from build123d import *

# Parameters (mm, degrees)
SKETCH1_W           = 72.136
SKETCH1_H           = 97.536
BOSS_EXTRUDE1_DEPTH = 6.35
CUT_EXTRUDE4_REACH  = 123.479
SKETCH12_R          = 2.54
SKETCH13_R          = 1.27
CUT_EXTRUDE5_DEPTH  = 3.81


with BuildPart() as part:
    # Sketch1 → Boss-Extrude1 (new body)
    with BuildSketch(Plane.XY):
        with Locations((36.068, -48.768)):
            Rectangle(SKETCH1_W, SKETCH1_H)
    extrude(amount=BOSS_EXTRUDE1_DEPTH)

    # Sketch12 → Cut-Extrude4 (cut, up to next)
    with BuildSketch(Plane.XY.offset(6.35), mode=Mode.PRIVATE) as cut_extrude4_sk1:
        with Locations((3.048, -3.048)):
            Circle(SKETCH12_R)
    cut_extrude4_tool1 = extrude(cut_extrude4_sk1.sketch, amount=-CUT_EXTRUDE4_REACH, mode=Mode.PRIVATE) & part.part
    # Sketch12 → Cut-Extrude4 (cut, up to next)
    with BuildSketch(Plane.XY.offset(6.35), mode=Mode.PRIVATE) as cut_extrude4_sk2:
        with Locations((69.088, -3.048)):
            Circle(SKETCH12_R)
    cut_extrude4_tool2 = extrude(cut_extrude4_sk2.sketch, amount=-CUT_EXTRUDE4_REACH, mode=Mode.PRIVATE) & part.part
    # Sketch12 → Cut-Extrude4 (cut, up to next)
    with BuildSketch(Plane.XY.offset(6.35), mode=Mode.PRIVATE) as cut_extrude4_sk3:
        with Locations((69.088, -94.488)):
            Circle(SKETCH12_R)
    cut_extrude4_tool3 = extrude(cut_extrude4_sk3.sketch, amount=-CUT_EXTRUDE4_REACH, mode=Mode.PRIVATE) & part.part
    # Sketch12 → Cut-Extrude4 (cut, up to next)
    with BuildSketch(Plane.XY.offset(6.35), mode=Mode.PRIVATE) as cut_extrude4_sk4:
        with Locations((3.048, -94.488)):
            Circle(SKETCH12_R)
    cut_extrude4_tool4 = extrude(cut_extrude4_sk4.sketch, amount=-CUT_EXTRUDE4_REACH, mode=Mode.PRIVATE) & part.part
    add(cut_extrude4_tool1.solids().sort_by_distance((3.048, -3.048, 6.35))[0], mode=Mode.SUBTRACT)
    add(cut_extrude4_tool2.solids().sort_by_distance((69.088, -3.048, 6.35))[0], mode=Mode.SUBTRACT)
    add(cut_extrude4_tool3.solids().sort_by_distance((69.088, -94.488, 6.35))[0], mode=Mode.SUBTRACT)
    add(cut_extrude4_tool4.solids().sort_by_distance((3.048, -94.488, 6.35))[0], mode=Mode.SUBTRACT)

    # Sketch13 → Cut-Extrude5 (cut)
    with BuildSketch(Plane.XY.offset(6.35)):
        with Locations((12.7, -12.7)):
            Circle(SKETCH13_R)
        with Locations((59.436, -12.7)):
            Circle(SKETCH13_R)
    extrude(amount=-CUT_EXTRUDE5_DEPTH, mode=Mode.SUBTRACT)


solid = part.part
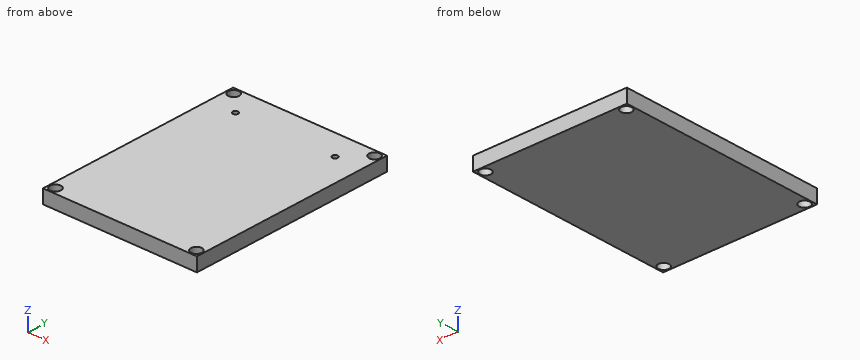
Geometry check sheet. Reference: the model listing, model coordinates, mm. Coordinates: 2 decimals unless noted, no trailing zeros. Order: outer loops, then holes, each group sorted by start corner. A loop starts at its lowest first (then second) coordinate and runs counter-clockwise, first axis right, second up. Notation, with made-up numbers: (-6, 60.25) - (40, 60.25) arc R10 ccw to (40, 68.25) - close; hole circle Ø5 at (34.25, 73). An arc over 180 degrees is marked (long way). Answer in a Markdown table with one row per item. Add a question column.
1) Cross-section at B-B, the plane x = 12.7. Record the cut outline in (y, z).
2) Material ranges on line 1 along Y through (x, z) = (12.7, 5.4); line 2 along X through (y, z) = (-92.5, 3), recorded low to high. Write a range as [from, to].
3) Cross-section at A-A, the plane y = -12.7. Record the cut outline in (x, z), then the cut area to 3 significant figures.
4) Gauge pin test, flat ends, axial feed: P1, Ø3, axis at x = 59.436, y = -12.7, coming from the +Z side; P2, Ø2, axis at x = 12.7, y = -12.7, coming from the +Z side. Record the tip position at first contact, or that the pin passes through.
Check result:
| question | item | result |
|---|---|---|
| 1 | outline | (-97.54, 0) - (0, 0) - (0, 6.35) - (-11.43, 6.35) - (-11.43, 2.54) - (-13.97, 2.54) - (-13.97, 6.35) - (-97.54, 6.35) - close |
| 2 | line 1 | y = [-97.54, -13.97], [-11.43, 0] |
| 2 | line 2 | x = [0, 1.47], [4.63, 67.51], [70.67, 72.14] |
| 3 | outline | (0, 0) - (72.14, 0) - (72.14, 6.35) - (60.71, 6.35) - (60.71, 2.54) - (58.17, 2.54) - (58.17, 6.35) - (13.97, 6.35) - (13.97, 2.54) - (11.43, 2.54) - (11.43, 6.35) - (0, 6.35) - close |
| 3 | area | 439 mm² |
| 4 | P1 | stops at z = 6.35 |
| 4 | P2 | stops at z = 2.54 |
